```python
from build123d import *

# Parameters (mm, degrees)
ESBO_O1_W                  = 47.3
ESBO_O1_H                  = 28
RESSALTO_EXTRUS_O1_DEPTH   = 55.6
CORTE_EXTRUS_O1_DEPTH      = 67.593411836
CORTE_EXTRUS_O2_DEPTH      = 67.593411836
CORTE_EXTRUS_O3_DEPTH      = 75.327989345
CORTE_EXTRUS_O3_DEPTH_BACK = 5.6
ESBO_O4_R                  = 5
ESBO_O5_R                  = 4
CORTE_EXTRUS_O6_DEPTH      = 5.6
FILETE1_R                  = 14
FILETE2_R                  = 14
ESBO_O6_R                  = 5
CORTE_EXTRUS_O7_DEPTH      = 5.6


with BuildPart() as part:
    # Esboço1 → Ressalto-extrusão1 (new body)
    with BuildSketch(Plane.XY):
        Rectangle(ESBO_O1_W, ESBO_O1_H)
    extrude(amount=RESSALTO_EXTRUS_O1_DEPTH)

    # Esboço2 → Corte-extrusão1 (cut, through all)
    with BuildSketch(Plane(origin=(0, 14, 0), x_dir=(1, 0, 0), z_dir=(0, 1, 0))):
        Polygon((-23.65, -27.6), (-23.65, 0), (-14, 0), align=None)
        Polygon((14, 0), (23.65, 0), (23.65, -27.6), align=None)
    extrude(amount=-CORTE_EXTRUS_O1_DEPTH, mode=Mode.SUBTRACT)

    # Esboço3 → Corte-extrusão2 (cut, through all)
    with BuildSketch(Plane(origin=(0, 14, 0), x_dir=(1, 0, 0), z_dir=(0, 1, 0))):
        Polygon((-21.15, -28.02444916), (-21.15, -55.6), (21.15, -55.6), (21.15, -28.02444916), (12.225690783, -2.5), (-12.225690783, -2.5), align=None)
    extrude(amount=-CORTE_EXTRUS_O2_DEPTH, mode=Mode.SUBTRACT)

    # Esboço4 → Corte-extrusão3 (cut, two sides: drawn at the far end of the back side and taken through both)
    with BuildSketch(Plane(origin=(23.65, 0, 0), x_dir=(0, 0, -1), z_dir=(1, 0, 0)).offset(-CORTE_EXTRUS_O3_DEPTH_BACK)):
        with Locations(Location((-41.6, 0, 0), (0, 0, 270))):
            Circle(ESBO_O4_R)
    extrude(amount=CORTE_EXTRUS_O3_DEPTH + CORTE_EXTRUS_O3_DEPTH_BACK, mode=Mode.SUBTRACT)

    # Esboço5 → Corte-extrusão6 (cut)
    with BuildSketch(Plane.ZY.offset(23.65)):
        with Locations(Location((41.6, 0, 0), (0, 0, 270))):
            Circle(ESBO_O5_R)
    extrude(amount=-CORTE_EXTRUS_O6_DEPTH, mode=Mode.SUBTRACT)

    # Filete1
    filete1_edges = [part.edges().sort_by_distance(p)[0] for p in [
        (-22.4, -14, 55.6),
        (-22.4, 14, 55.6),
    ]]
    fillet(filete1_edges, radius=FILETE1_R - 0.0001)  # a hair under: the kernel refuses the full size

    # Filete2
    filete2_edges = [part.edges().sort_by_distance(p)[0] for p in [
        (22.4, -14, 55.6),
        (22.4, 14, 55.6),
    ]]
    fillet(filete2_edges, radius=FILETE2_R - 0.0001)  # a hair under: the kernel refuses the full size

    # Esboço6 → Corte-extrusão7 (cut)
    with BuildSketch(Plane(origin=(0, 0, 0), x_dir=(-1, 0, 0), z_dir=(0, 0, -1))):
        Circle(ESBO_O6_R)
    extrude(amount=-CORTE_EXTRUS_O7_DEPTH, mode=Mode.SUBTRACT)


solid = part.part
```
Build history of the part. All positions in model axes, mm. A direction names the side the tool comes from. Round coordinates to 2 decimals unless told otherwise and drop trailing zeros. Write each loop counter-clockwise with the first axis right and the second up, starting at its lowest first coordinate (ties: lowest second). Pieces come first, ordered by that corner, then holes. Notation, with made-up numbers: (82.25, 11.5) - (88.25, 11.5) arc R30 ccw to (88.25, 49.5) - close; hole circle Ø9 at (49.25, 32.25). An arc over 180 degrees is marked (long way). Write each question's results on one line, items separated by ' | '. Start each with the question number.
Item 1: Saw through at A-A (x = 0). Write the cut outline in (y, z), and give its area (3 significant figures).
Item 2: Saw through at C-C (y = 9.5). Write the cut outline in (x, z).
Item 3: Drop flat-ended pins along their axis: P1, Ø12, axis at x = -5, y = 8.5, coming from the +Z side; P2, Ø3, axis at y = -5, z = 23, coming from the -X side; P3, Ø5, axis at y = -7, z = 24, coming from the +X side. Give the stop position or say it passes through.
Item 4: Saw through at D-D (x = 8). Write the cut outline in (y, z), and give its area (3 significant figures).
Item 5: Saw through at B-B (z = 25). Write the cut outline in (x, y), and give its area (3 significant figures).
Item 6: Which spindle directions (+Z, -Z, +X, -X, +Y, -Y) get a long thin tool onto all of the face, cutting with end or side? Do faces 4 (the face through (-21.15, -2.9, 38.6)), 5 (the face through (22.38, 1.08, 46.48)), 6 (the face through (-22.417, -2.15, 44.973)). Say none if no direction does.
Item 7: Wall check: L1, parallel to X at y = -12.25, z = 39.5; L2, parallel to Y at x = 0, z = 1.7. Give the ranges that are in metal, low to high. Write a range as [from, to].
Item 8: Mould opens along X. For faces 1 (the face through (-23.65, 3, 38)), 2 (the face through (1.08, -4.88, 1.23)), 3 (the face through (22.4, -10, 51.4)) say: pulls with the +X half, pulls with the -X half, needs draft (parallel to the pull), parting line crosses it, or undercut.
Results are:
1) outline: (-14, 0) - (-5, 0) - (-5, 2.5) - (-14, 2.5) - close; (5, 0) - (14, 0) - (14, 2.5) - (5, 2.5) - close | area: 45.0 mm²
2) outline: (-23.65, 27.6) - (-14, 0) - (14, 0) - (23.65, 27.6) - (23.65, 51.88) - (21.15, 51.88) - (21.15, 28.02) - (12.23, 2.5) - (-12.23, 2.5) - (-21.15, 28.02) - (-21.15, 51.88) - (-23.65, 51.88) - close
3) P1: stops at z = 2.5 | P2: stops at x = -22.57 | P3: stops at x = 23.27
4) outline: (-14, 0) - (14, 0) - (14, 2.5) - (-14, 2.5) - close | area: 70.0 mm²
5) outline: (-22.74, -14) - (-20.09, -14) - (-20.09, 14) - (-22.74, 14) - close; (20.09, -14) - (22.74, -14) - (22.74, 14) - (20.09, 14) - close | area: 148 mm²
6) face 4: +Z, +Y, -Y | face 5: +X | face 6: +X, -X
7) L1: x = [-23.65, -21.15], [21.15, 23.65] | L2: y = [-14, -5], [5, 14]
8) face 1: pulls with the -X half | face 2: undercut | face 3: needs draft
